Verification items for the finished model (mm, model axes). Face numbers are marked on the shaded views. A direction names the side the tool comes from. Give positions to 0.01 mm unless a question says otherwise; leave off trailing zeros. Write each loop counter-clockwise with the first axis right and the second up, starting at its lowest first coordinate (ties: lowest second). Pieces come first, ordered by that corner, then holes. Notation, with made-up numbers: (2, 83) -> (12, 83) arc R8 ccw to (12, 94) -> close; hole circle Ø2 at (18, 7). An arc over 180 degrees is marked (long way). Use CSV: the item, a comma, the result in double quotes. Start each with the question number.
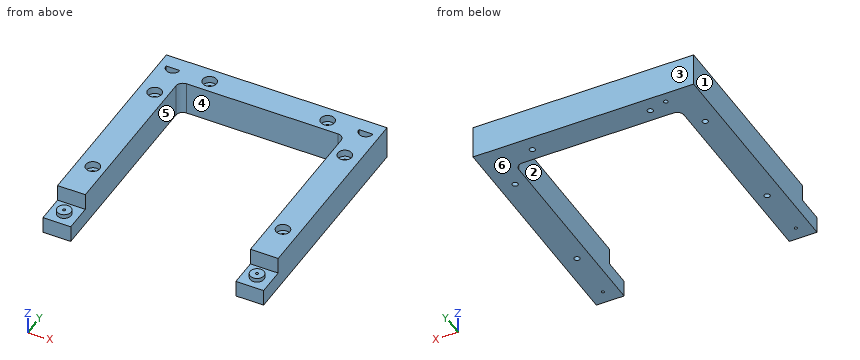
Autodesk Inventor part; units mm, degrees
ref_plane "YZ Plane" through (0, 0, 0) normal (1, 0, 0) x (0, 1, 0)
ref_plane "XZ Plane" through (0, 0, 0) normal (0, 1, 0) x (-1, 0, 0)
ref_plane "XY Plane" through (0, 0, 0) normal (0, 0, 1) x (1, 0, 0)
sketch "Sketch1" plane through (0, 0, 0) normal (0, 0, 1) x (1, 0, 0)
  line L0 (-79.5, -159.5) -> (79.5, -159.5)
  line L1 (79.5, -159.5) -> (79.5, 159.5)
  line L2 (79.5, 159.5) -> (-79.5, 159.5)
  line L3 (-79.5, 159.5) -> (-79.5, -159.5)
  line L4 (-79.5, -159.5) -> (79.5, 159.5) construction
  line L5 (79.5, -159.5) -> (-79.5, 159.5) construction
  line L6 (-59.5, -139.5) -> (59.5, -139.5)
  line L7 (59.5, -139.5) -> (59.5, 139.5)
  line L8 (59.5, 139.5) -> (-59.5, 139.5)
  line L9 (-59.5, 139.5) -> (-59.5, -139.5)
  line L10 (-59.5, -139.5) -> (59.5, 139.5) construction
  line L11 (59.5, -139.5) -> (-59.5, 139.5) construction
  circle A0 centre (68.5, -122.5) radius 1
  circle A1 centre (42.5, -148.5) radius 1
  circle A2 centre (68.5, -37.5) radius 1
  circle A3 centre (-68.5, -37.5) radius 1
  circle A4 centre (-68.5, -122.5) radius 1
  circle A5 centre (-42.5, -148.5) radius 1
  circle A6 centre (68.5, 122.5) radius 1
  circle A7 centre (42.5, 148.5) radius 1
  circle A8 centre (68.5, 37.5) radius 1
  circle A9 centre (-68.5, 37.5) radius 1
  circle A10 centre (-68.5, 122.5) radius 1
  circle A11 centre (-42.5, 148.5) radius 1
  circle A12 centre (-42.5, 148.5) radius 2
  circle A13 centre (-68.5, 122.5) radius 2
  circle A14 centre (42.5, 148.5) radius 2
  circle A15 centre (68.5, 122.5) radius 2
  circle A16 centre (68.5, 37.5) radius 2
  circle A17 centre (-68.5, 37.5) radius 2
  circle A18 centre (-68.5, -37.5) radius 2
  circle A19 centre (-68.5, -122.5) radius 2
  circle A20 centre (-42.5, -148.5) radius 2
  circle A21 centre (42.5, -148.5) radius 2
  circle A22 centre (68.5, -122.5) radius 2
  circle A23 centre (68.5, -37.5) radius 2
  point P0 (0, 0)
  dimension "d0" = 159
  dimension "d1" = 319
  dimension "d2" = 119
  dimension "d3" = 279
  dimension "d4" = 2
  dimension "d5" = 11
  dimension "d6" = 37
  dimension "d7" = 2
  dimension "d8" = 11
  dimension "d9" = 37
  dimension "d10" = 2
  dimension "d11" = 11
  dimension "d12" = 122
  dimension "d13" = 4
  dimension "d14" = 4
  dimension "d15" = 4
  dimension "d16" = 4
  dimension "d17" = 4
  dimension "d18" = 4
  dimension "d19" = 4
  dimension "d20" = 4
  dimension "d21" = 4
  dimension "d22" = 4
  dimension "d23" = 4
  dimension "d24" = 4
extrude "Extrusion1" add sketch "Sketch1" along normal blind 24 contours L3 L2 L1 L0
sketch "Sketch2" plane through (0, 0, 24) normal (0, 0, 1) x (1, 0, 0)
  circle A0 centre (42.5, -148.5) radius 2
  circle A1 centre (42.5, -148.5) radius 5
  circle A2 centre (68.5, -122.5) radius 2
  circle A3 centre (68.5, -122.5) radius 5
  circle A4 centre (68.5, -37.5) radius 2
  circle A5 centre (68.5, -37.5) radius 5
  circle A6 centre (-42.5, -148.5) radius 5
  circle A7 centre (-68.5, -122.5) radius 5
  circle A8 centre (-68.5, -37.5) radius 5
  circle A9 centre (-68.5, 37.5) radius 5
  circle A10 centre (-68.5, 122.5) radius 5
  circle A11 centre (-42.5, 148.5) radius 5
  circle A12 centre (42.5, 148.5) radius 5
  circle A13 centre (68.5, 122.5) radius 5
  circle A14 centre (68.5, 37.5) radius 5
  point P0 (0, 0)
  dimension "d27" = 10
  dimension "d28" = 10
  dimension "d29" = 10
extrude "Extrusion2" cut sketch "Sketch2" against normal blind 5
sketch "Sketch3" plane through (0, 0, 24) normal (0, 0, 1) x (1, 0, 0)
  circle A0 centre (-69.5, 149.5) radius 5
  line L0 (79.5, 159.5) -> (-79.5, 159.5)
  line L1 (-79.5, 159.5) -> (-79.5, -159.5)
  line L2 (0, 115.3552) -> (0, 76.8376)
  circle A1 centre (69.5, 149.5) radius 5
  point P0 (0, 0)
  dimension "d32" = 10
  dimension "d33" = 10
  dimension "d34" = 10
extrude "Extrusion3" cut sketch "Sketch3" against normal blind 11.5
sketch "Sketch4" plane through (0, 0, 24) normal (0, 0, 1) x (1, 0, 0)
  circle A0 centre (-69.5, 149.5) radius 5
  line L0 (-74.5, 149.5) -> (-64.5, 149.5)
  circle A1 centre (69.5, 149.5) radius 5
  line L1 (64.5, 149.5) -> (74.5, 149.5)
  point P0 (0, 0)
extrude "Extrusion4" add sketch "Sketch4" against normal blind 5.75 contours L0 A0 | L1 A1 picked at (-70.091, 152.6074) picked at (68.909, 152.6074)
sketch "Sketch5" plane through (0, 0, 0) normal (0, 0, -1) x (-1, 0, 0)
  circle A0 centre (-55.5, -152) radius 1.5
  line L0 (79.5, -159.5) -> (-79.5, -159.5)
  line L1 (-79.5, -159.5) -> (-79.5, 159.5)
  circle A1 centre (55.5, 152) radius 1.5
  line L2 (-79.5, 159.5) -> (79.5, 159.5)
  line L3 (79.5, 159.5) -> (79.5, -159.5)
  point P0 (0, 0)
  dimension "d39" = 3
  dimension "d40" = 7.5
  dimension "d41" = 24
  dimension "d42" = 3
  dimension "d43" = 7.5
  dimension "d44" = 24
extrude "Extrusion5" cut sketch "Sketch5" against normal blind 5 contours A0 | A1
sketch "Sketch6" plane through (0, 0, 24) normal (0, 0, 1) x (1, 0, 0)
  line L0 (-79.5, -159.5) -> (79.5, -159.5)
  line L1 (79.5, -159.5) -> (79.5, 159.5)
  point P0 (0, 0)
sketch "Sketch7" plane through (0, 0, 24) normal (0, 0, 1) x (1, 0, 0)
  point P0 (0, 0)
sketch "Sketch8" plane through (0, 0, 24) normal (0, 0, 1) x (1, 0, 0)
  line L0 (-16.5, -124.5) -> (-16.5, -58.5)
  line L1 (-79.5, -159.5) -> (79.5, -159.5)
  line L2 (79.5, -159.5) -> (79.5, 159.5)
  line L3 (59.5, -139.5) -> (59.5, 139.5)
  line L4 (-16.5, -58.5) -> (59.5, -58.5)
  line L5 (-16.5, -124.5) -> (59.5, -124.5)
  line L6 (59.5, 139.5) -> (59.5, -139.5)
  point P0 (0, 0)
sketch "Sketch9" plane through (0, 0, 24) normal (0, 0, 1) x (1, 0, 0)
  point P0 (0, 0)
sketch "Sketch10" plane through (0, 0, 24) normal (0, 0, 1) x (1, 0, 0)
  point P0 (0, 0)
sketch "Sketch11" plane through (0, 0, 24) normal (0, 0, 1) x (1, 0, 0)
  point P0 (0, 0)
sketch "Sketch12" plane through (0, 0, 24) normal (0, 0, 1) x (1, 0, 0)
  point P0 (0, 0)
extrude "Extrusion6" add sketch "Sketch8" against normal blind 2
fillet "Fillet1" radius 5 6 edges at (59.5, -139.5, 12) (59.5, -58.5, 23) (-59.5, -139.5, 12) (59.5, -124.5, 23) (-59.5, 139.5, 12) (59.5, 139.5, 12)
fillet "Fillet2" radius 2 2 edges at (-16.5, -58.5, 23) (-16.5, -124.5, 23)
sketch "Sketch13" plane through (0, 0, 24) normal (0, 0, 1) x (1, 0, 0)
  point P0 (0, 0)
sketch "Sketch14" plane through (0, 0, 24) normal (0, 0, 1) x (1, 0, 0)
  circle A0 centre (-11.8564, -120.5) radius 0.5
  circle A1 centre (-11.8564, -62.5) radius 0.5
  circle A2 centre (37.1436, -120.5) radius 0.5
  circle A3 centre (37.1436, -62.5) radius 0.5
  line L0 (-14.5, -124.5) -> (54.5, -124.5)
  point P0 (0, 0)
  dimension "d58" = 1
  dimension "d59" = 1
  dimension "d60" = 58
  dimension "d61" = 1
  dimension "d62" = 1
  dimension "d63" = 49
  dimension "d64" = 49
  dimension "d65" = 4
extrude "Extrusion7" cut sketch "Sketch14" against normal blind 20
fillet "Fillet3" radius 5 1 edges at (59.5, -91.5, 22)
sketch "Sketch15" plane through (0, 0, 22) normal (0, 0, -1) x (-1, 0, 0)
  circle A0 centre (-37.1436, -62.5) radius 0.5
  circle A1 centre (-37.1436, -120.5) radius 0.5
  circle A2 centre (-37.1436, -62.5) radius 0.5
  circle A3 centre (-37.1436, -62.5) radius 4
  circle A4 centre (11.8564, -62.5) radius 0.5
  circle A5 centre (11.8564, -62.5) radius 4
  circle A6 centre (11.8564, -120.5) radius 0.5
  circle A7 centre (11.8564, -120.5) radius 4
  circle A8 centre (-37.1436, -120.5) radius 0.5
  circle A9 centre (-37.1436, -120.5) radius 4
  point P0 (0, 0)
  dimension "d71" = 8
  dimension "d72" = 8
  dimension "d73" = 8
  dimension "d74" = 8
extrude "Extrusion8" add sketch "Sketch15" along normal blind 2
sketch "Sketch17" plane through (-79.5, -159.5, 0) normal (0, -1, 0) x (1, 0, 0)
  line L0 (93, 24) -> (113, 24)
  line L1 (113, 24) -> (113, 14)
  line L2 (113, 14) -> (93, 14)
  line L3 (93, 14) -> (93, 24)
  line L4 (0, 24) -> (159, 24)
  line L5 (0, 0) -> (0, 24)
  point P0 (79.5, 0)
  dimension "d83" = 20
  dimension "d84" = 10
  dimension "d85" = 93
extrude "Extrusion10" cut sketch "Sketch17" against normal blind 21
fillet "Fillet4" radius 2 4 edges at (13.5, -149.5, 14) (13.5, -149.5, 24) (33.5, -149.5, 24) (33.5, -149.5, 14)
sketch "Sketch18" plane through (0, 0, 24) normal (0, 0, 1) x (1, 0, 0)
  point P0 (0, 0)
sketch "Sketch19" plane through (79.5, -159.5, 0) normal (1, 0, 0) x (0, 0, -1)
  line L0 (-24, 169.5) -> (-12, 169.5)
  line L1 (-12, 169.5) -> (-12, 149.5)
  line L2 (-12, 149.5) -> (0, 149.5)
  line L3 (-24, 319) -> (-24, 0)
  point P0 (0, 159.5)
  dimension "d89" = 12
  dimension "d90" = 20
  dimension "d91" = 12
split body "Split1" sketch "Sketch19" result one side removed curves L0 L1 L2 removed pieces at (4.5717, -81.9705, 23.5)
sketch "Sketch20" plane through (59.5, 10, 12) normal (0, 0, 1) x (1, 0, 0)
  circle A0 centre (-129, -10) radius 5
  line L0 (-119, 0) -> (-119, -20)
  line L1 (-139, -20) -> (-119, -20)
  line L2 (-59.5, -10) -> (-59.5, -28.6387)
  circle A1 centre (10, -10) radius 5
  dimension "d93" = 10
  dimension "d94" = 10
  dimension "d95" = 10
extrude "Extrusion13" add sketch "Sketch20" along normal blind 3
sketch "Sketch22" plane through (-69.5, 0, 15) normal (0, 0, 1) x (1, 0, 0)
  circle A0 centre (0, 0) radius 1
  circle A1 centre (139, 0) radius 1
  point P0 (69.5, 0)
  dimension "d103" = 2
extrude "Extrusion14" cut sketch "Sketch22" against normal blind 33
properties part number "led_matrix_frame_upper"
(1) Thickness scan on line 1 (Y direction, x = -42.5, z = 21.75); line 2 (Y direction, x = -65, z = 23); line 3 (Y direction, x = -69, z = 20.5). Record the ranges inside material, lowest first. Write a range as from..to.
(2) Section check B-B on z = 21.25. Give the number of separate pieces and of enclosed holes in the cut face, then the cut area to 3 significant figures.
(3) Section check C-C on y = 37.5. Record the cut outline in (x, z).
(4) Draft check along X on the marked faces 1, 2, 3 and 4. Enter one of: released by +X, released by -X, zero draft, split by the parting line, or undercut.
(5) Section check D-D on y = 20. Record the cut outline in (x, z).
(6) Set-up check for the marked faces 5 and 6: record each of +Z, -Z, +X, -X, +Y, -Y from which the full face is reachable in a straight line by a thin tool's end or side.
(7) Go/stop test with flat-tipped pins: pin 1 (3 mm diameter, centred on x = 39, z = 4, fed in from -Y); pin 2 (5 mm diameter, centred on x = -68.5, y = 37.5, fed in from +Z); pin 3 (2.5 mm diameter, centred on x = -55.5, y = 152, fed in from -Z). Record where each tip stops, or that it passes through.
(8) Section check A-A on x = -42.5. Record the cut outline in (y, z), then the cut area to 3 significant figures.
Data:
1,line 1,"y = 139.5..143.5, 153.5..159.5"
1,line 2,"y = 10..33.93, 41.07..118.93, 126.07..147.32, 149.5..159.5"
1,line 3,"y = 10..32.53, 42.47..117.53, 127.47..144.53, 149.5..159.5"
2,separate pieces,"1"
2,enclosed holes,"8"
2,area,"7,820 mm2"
3,outline,"(-79.5, 0) -> (-70.5, 0) -> (-70.5, 19) -> (-73.5, 19) -> (-73.5, 24) -> (-79.5, 24) -> close; (-66.5, 0) -> (-59.5, 0) -> (-59.5, 24) -> (-63.5, 24) -> (-63.5, 19) -> (-66.5, 19) -> close; (59.5, 0) -> (66.5, 0) -> (66.5, 19) -> (63.5, 19) -> (63.5, 24) -> (59.5, 24) -> close; (70.5, 0) -> (79.5, 0) -> (79.5, 24) -> (73.5, 24) -> (73.5, 19) -> (70.5, 19) -> close"
4,face 1,"released by -X"
4,face 2,"undercut"
4,face 3,"zero draft"
4,face 4,"undercut"
5,outline,"(-79.5, 0) -> (-59.5, 0) -> (-59.5, 24) -> (-79.5, 24) -> close; (59.5, 0) -> (79.5, 0) -> (79.5, 24) -> (59.5, 24) -> close"
6,face 5,"+Z, -Z, -Y"
6,face 6,"-Z, +X, -X, +Y, -Y"
7,pin 1,"stops at y = 139.5"
7,pin 2,"stops at z = 19"
7,pin 3,"stops at z = 5"
8,outline,"(139.5, 0) -> (146.5, 0) -> (146.5, 19) -> (143.5, 19) -> (143.5, 24) -> (139.5, 24) -> close; (150.5, 0) -> (159.5, 0) -> (159.5, 24) -> (153.5, 24) -> (153.5, 19) -> (150.5, 19) -> close"
8,area,"354 mm2"
